Check sheet for the modelled part. Datum: model origin and axes. Units: mm. A direction names the side the tool comes from. Coordinates: 2 decimals unless noted, no trailing zeros. Order: outer loops, then holes, each group sorted by start corner. A loop starts at its lowest first (then second) coordinate and runs counter-clockwise, first axis right, second up.
Autodesk Inventor part; units mm, degrees
ref_plane "YZ Plane" through (0, 0, 0) normal (1, 0, 0) x (0, 1, 0)
ref_plane "XZ Plane" through (0, 0, 0) normal (0, 1, 0) x (-1, 0, 0)
ref_plane "XY Plane" through (0, 0, 0) normal (0, 0, 1) x (1, 0, 0)
sketch "Sketch1" plane through (0, 0, 0) normal (1, 0, 0) x (0, 1, 0)
  line L0 (0, 0) -> (0, -31.75)
  line L1 (0, 0) -> (173.355, 0)
  line L2 (0, 0) -> (173.355, 0)
  line L3 (173.355, 0) -> (173.355, -31.75)
  line L4 (173.355, -31.75) -> (0, -31.75)
  line L5 (0, -31.75) -> (0, 0)
  line L6 (0, -15.875) -> (6.35, -15.875)
  line L7 (173.355, -15.875) -> (167.005, -15.875)
  arc A0 (155.0924, -27.7876) -> (155.0924, -3.9624) centre (155.0924, -15.875) ccw
  line L8 (155.0924, -3.9624) -> (30.9626, -3.9624)
  line L9 (30.9626, -27.7876) -> (155.0924, -27.7876)
  arc A1 (30.9626, -3.9624) -> (30.9626, -27.7876) centre (30.9626, -15.875) ccw
  dimension "d0" = 31.75
  dimension "d1" = 173.355
  dimension "d2" = 6.35
  dimension "d3" = 6.35
extrude "Extrusion1" add sketch "Sketch1" against normal blind 118.11
sketch "Sketch2" plane through (0, 0, 0) normal (0, 0, 1) x (1, 0, 0)
  line L0 (0, 173.355) -> (0, 0)
  line L1 (0, 173.355) -> (-118.11, 173.355)
  line L2 (-118.11, 0) -> (-118.11, 173.355)
  line L3 (0, 0) -> (-118.11, 0)
  line L4 (-6.35, 6.35) -> (-6.35, 167.005)
  line L5 (-6.35, 167.005) -> (-111.76, 167.005)
  line L6 (-111.76, 167.005) -> (-111.76, 6.35)
  line L7 (-111.76, 6.35) -> (-6.35, 6.35)
  dimension "d9" = 6.35
extrude "Extrusion2" cut sketch "Sketch2" against normal blind 118.11 contours L7 L6 L5 L4
sketch "Sketch3" plane through (0, 0, 0) normal (0, 0, 1) x (1, 0, 0)
  point P0 (0, 0)
sketch "Sketch4" plane through (0, 0, 0) normal (0, 0, 1) x (1, 0, 0)
  line L0 (-111.76, 167.005) -> (-6.35, 167.005)
  circle A0 centre (-59.055, 140.6525) radius 26.3525
  line L1 (-111.76, 30.9626) -> (-111.76, 155.0924)
  line L2 (-111.76, 114.3) -> (-6.35, 114.3)
  line L3 (-6.35, 114.3) -> (-6.35, 167.005)
  line L4 (-6.35, 167.005) -> (-111.76, 167.005)
  line L5 (-111.76, 167.005) -> (-111.76, 114.3)
  point P0 (0, 0)
  point P1 (-59.055, 167.005)
  point P2 (-59.055, 114.3)
extrude "Extrusion3" add sketch "Sketch4" against normal blind 31.75 contours L0 A0 L2 L1 L5 | L0 L3 L2 A0
sketch "Sketch5" plane through (0, 0, 0) normal (1, 0, 0) x (0, 0, -1)
  line L0 (0, 173.355) -> (0, 0)
  line L1 (0, 0) -> (31.75, 0)
  line L2 (31.75, 0) -> (31.75, 173.355)
  line L3 (31.75, 173.355) -> (0, 173.355)
  arc A0 (27.7876, 155.0924) -> (3.9624, 155.0924) centre (15.875, 155.0924) ccw
  line L4 (27.7876, 155.0924) -> (27.7876, 30.9626)
  arc A1 (3.9624, 30.9626) -> (27.7876, 30.9626) centre (15.875, 30.9626) ccw
  line L5 (3.9624, 30.9626) -> (3.9624, 155.0924)
extrude "Extrusion4" cut sketch "Sketch5" against normal through all contours L4 A1 L5 A0
sketch "Sketch6" plane through (0, 0, -31.75) normal (0, -1, 0) x (1, 0, 0)
  line L0 (-118.11, 3.9624) -> (-118.11, 27.7876)
  line L1 (0, 27.7876) -> (0, 3.9624)
  line L2 (-81.0991, 27.7876) -> (-118.11, 27.7876)
  line L3 (-99.6046, 27.7876) -> (-18.2626, 27.7876)
  line L4 (-6.35, 3.9624) -> (-59.055, 3.9624)
  line L5 (-18.2626, 3.9624) -> (-99.6046, 3.9624)
  line L6 (-81.0991, 3.9624) -> (-118.11, 3.9624)
  line L7 (0, 0) -> (0, 31.75)
  line L8 (0, 15.875) -> (-12.7, 15.875)
  line L9 (-118.11, 0) -> (-118.11, 31.75)
  line L10 (-118.11, 15.875) -> (-105.41, 15.875)
  arc A0 (-24.6126, 3.9624) -> (-24.6126, 27.7876) centre (-24.6126, 15.875) ccw
  arc A1 (-93.4974, 27.7876) -> (-93.4974, 3.9624) centre (-93.4974, 15.875) ccw
  dimension "d21" = 12.7
  dimension "d22" = 12.7
extrude "Extrusion5" cut sketch "Sketch6" against normal blind 31.75 contours A1 L2 L3 A0 L4 L5
sketch "Sketch7" plane through (0, 173.355, 0) normal (0, 1, 0) x (1, 0, 0)
  line L0 (-24.6126, 3.9624) -> (-93.4974, 3.9624)
  line L1 (-93.4974, 27.7876) -> (-24.6126, 27.7876)
  arc A0 (-93.4974, 27.7876) -> (-93.4974, 3.9624) centre (-93.4974, 15.875) ccw
  arc A1 (-24.6126, 3.9624) -> (-24.6126, 27.7876) centre (-24.6126, 15.875) ccw
  point P0 (0, 0)
extrude "Extrusion6" cut sketch "Sketch7" against normal blind 31.75
sketch "Sketch8" plane through (0, 0, 0) normal (0, 0, 1) x (1, 0, 0)
  line L0 (-111.76, 6.35) -> (-111.76, 114.3)
  line L1 (-111.76, 114.3) -> (-59.055, 114.3)
  circle A0 centre (-59.055, 140.6525) radius 26.3525
  line L2 (-59.055, 114.3) -> (-6.35, 114.3)
  line L3 (-6.35, 114.3) -> (-6.35, 6.35)
  line L4 (-6.35, 6.35) -> (-111.76, 6.35)
  line L5 (0, 173.355) -> (0, 0)
  line L6 (0, 173.355) -> (-118.11, 173.355)
  line L7 (-118.11, 0) -> (-118.11, 173.355)
  line L8 (0, 0) -> (-118.11, 0)
  line L9 (-59.055, 120.65) -> (-118.11, 120.65)
  line L10 (-118.11, 120.65) -> (-118.11, 0)
  line L11 (-118.11, 0) -> (0, 0)
  line L12 (0, 0) -> (0, 120.65)
  line L13 (0, 120.65) -> (-59.055, 120.65)
  line L14 (-111.76, 167.005) -> (-6.35, 167.005)
  line L15 (-6.35, 167.005) -> (-6.35, 6.35)
  line L16 (-6.35, 6.35) -> (-111.76, 6.35)
  line L17 (-111.76, 6.35) -> (-111.76, 167.005)
  circle A1 centre (-59.055, 140.6525) radius 32.7025
  point P0 (-39.6901, 167.005)
  point P1 (-33.1831, 120.65)
  point P2 (-6.35, 120.65)
  point P3 (-84.9269, 120.65)
  point P4 (-78.4199, 167.005)
  point P5 (-111.76, 120.65)
  dimension "d27" = 6.35
  dimension "d28" = 6.35
  dimension "d29" = 6.35
extrude "Extrusion7" cut sketch "Sketch8" against normal through all contours L17 L14 A1 L9 | L13 A1 L14 L15
properties part number "box rim big"
(1) Cross-section at D-D (y = 157.5). Count the separate pieces of the cut face and the enclosed holes in it, and give its area (3 significant figures).
Filled in:
separate pieces: 8
enclosed holes: 0
area: 230 mm2
(2) Release check for a two-part mould opening along Y. For faces 1 (the flat face through (-41, 118, 0)), 2 (the flat face through (-76, 118, -3.962)), 3 (the flat face through (-58, 0, -2)), 4 (the flat face through (-33, 114.3, -2)) record: +Y half, -Y half, draft (parallel to the pull), parting line (faces both ways), or undercut.
Filled in:
face 1: draft
face 2: undercut
face 3: -Y half
face 4: undercut
(3) Cross-section at C-C (z = -25). Enter the section's corners in (x, y) (3 decimals), and give its area (3 significant figures).
Filled in:
outline: (-118.11, 0) - (-101.155, 0) - (-101.155, 6.35) - (-111.76, 6.35) - (-111.76, 23.305) - (-118.11, 23.305) - close; (-118.11, 162.75) - (-111.76, 162.75) - (-111.76, 167.005) - (-101.155, 167.005) - (-101.155, 173.355) - (-118.11, 173.355) - close; (-16.955, 0) - (0, 0) - (0, 23.305) - (-6.35, 23.305) - (-6.35, 6.35) - (-16.955, 6.35) - close; (-16.955, 167.005) - (-6.35, 167.005) - (-6.35, 162.75) - (0, 162.75) - (0, 173.355) - (-16.955, 173.355) - close
area: 700 mm2
(4) Cross-section at B-B (x = -57). Enter the section's corners in (y, z) (3 decimals), and give its area (3 significant figures).
Filled in:
outline: (0, -31.75) - (6.35, -31.75) - (6.35, -27.788) - (0, -27.788) - close; (0, -3.962) - (6.35, -3.962) - (6.35, 0) - (0, 0) - close; (114.3, -31.75) - (114.38, -31.75) - (114.38, -27.788) - (114.3, -27.788) - close; (114.3, -3.962) - (114.38, -3.962) - (114.38, 0) - (114.3, 0) - close; (166.925, -31.75) - (173.355, -31.75) - (173.355, -27.788) - (166.925, -27.788) - close; (166.925, -3.962) - (173.355, -3.962) - (173.355, 0) - (166.925, 0) - close
area: 102 mm2
(5) Thickness scan on probe 1 along Y at (x, z) = (-110, -29) (3 decimals); probe 2 along Y at (x, z) = (-8, -10) (3 decimals); probe 3 along X at (y, z) = (12.5, -18). Record the ranges inside material, lowest first.
Filled in:
probe 1: y = 0 to 6.35, 114.3 to 120.65, 167.005 to 173.355
probe 2: y = 0 to 6.35, 167.005 to 173.355
probe 3: x = -118.11 to -111.76, -6.35 to 0
(6) Tool access check on faces 5 (the cylindrical face through (-3.131, 19.053, -15.613)), 6 (the flat face through (-86, 114.3, -2)), 7 (the flat face through (-60, 3, -3.962)), 8 (the flat face through (-45.7, 117.6, -27.788)), 9 (the flat face through (-41, 119, -31.75)). Record the directions out of +Z, -Z, +X, -X, +Y, -Y that give a thin tool (end or side, any length) a straight path to the whole face; none if there is none.
Filled in:
face 5: +X, -X
face 6: +Z, -Z
face 7: +Y, -Y
face 8: none
face 9: -Z, +X, -X, +Y, -Y
(7) Cross-section at A-A (y = 89). Enter the section's corners in (x, z).
Filled in:
outline: (-118.11, -31.75) - (-111.76, -31.75) - (-111.76, -27.79) - (-118.11, -27.79) - close; (-118.11, -3.96) - (-111.76, -3.96) - (-111.76, 0) - (-118.11, 0) - close; (-6.35, -31.75) - (0, -31.75) - (0, -27.79) - (-6.35, -27.79) - close; (-6.35, -3.96) - (0, -3.96) - (0, 0) - (-6.35, 0) - close
